from build123d import *

# Parameters (mm, degrees)
BOSS_EXTRUDE3_DEPTH = 12.7
SKETCH2_R           = 2.38125
CUT_EXTRUDE1_DEPTH  = 7.63575
SKETCH3_R           = 2.38125
CUT_EXTRUDE2_DEPTH  = 7.63575


with BuildPart() as part:
    # Sketch1 → Boss-Extrude3 (new body)
    with BuildSketch(Plane.XY):
        with BuildLine():
            Line((51.176153738, -2.63525), (68.859545977, -2.63525))
            Line((68.859545977, -2.63525), (68.859545977, -9.271))
            Line((68.859545977, -9.271), (56.159545977, -9.271))
            ThreePointArc((56.159545977, -9.271), (40.248267325, -40.248267325), (9.271, -56.159545977))
            Line((9.271, -56.159545977), (9.271, -68.956153738))
            Line((9.271, -68.956153738), (2.63525, -68.956153738))
            Line((2.63525, -68.956153738), (2.63525, -51.176153738))
            ThreePointArc((2.63525, -51.176153738), (36.234950351, -36.234950351), (51.176153738, -2.63525))
        make_face()
    extrude(amount=BOSS_EXTRUDE3_DEPTH)

    # Sketch2 → Cut-Extrude1 (cut, through all)
    with BuildSketch(Plane(origin=(9.271, 0, 0), x_dir=(0, 0, -1), z_dir=(1, 0, 0))):
        with Locations((-6.35, -62.606153738)):
            Circle(SKETCH2_R)
    extrude(amount=-CUT_EXTRUDE1_DEPTH, mode=Mode.SUBTRACT)

    # Sketch3 → Cut-Extrude2 (cut, through all)
    with BuildSketch(Plane.XZ.offset(9.271)):
        with Locations((62.509545977, 6.35)):
            Circle(SKETCH3_R)
    extrude(amount=-CUT_EXTRUDE2_DEPTH, mode=Mode.SUBTRACT)


solid = part.part
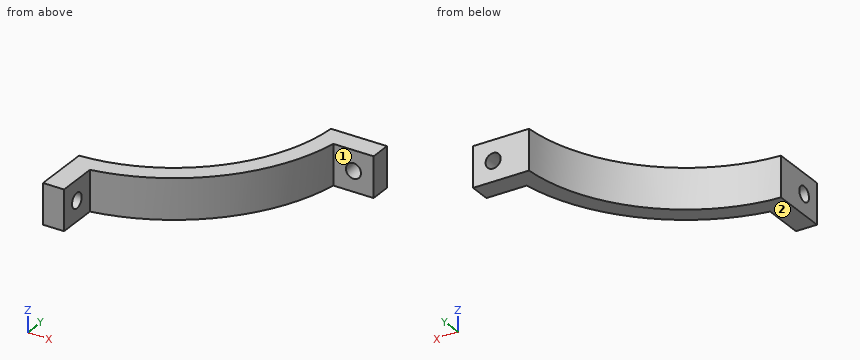
Could you check a few things on this model? Use its own coordinates, in mm. Face numbers are marked on the shaded views. A direction names the side the tool comes from. Coordinates: 2 decimals unless noted, no trailing zeros. Loops run counter-clockwise (first coordinate to the right, second up) from the corner with the lowest first, then second, coordinate; pieces in that order, holes last. Notation, with made-up numbers: (8.25, 82) -> (58.25, 82) arc R26 ccw to (58.25, 113) -> close; hole circle Ø1 at (88.25, 5). An arc over 180 degrees is marked (long way). Answer in a Markdown table with one row per item.
(1) If I drill on probe 1 along Y at (x, z) = (5.5, 6.35); probe 2 along X at (y, z) = (-56.5, 4.5); probe 3 along Y at (x, z) = (24, 11.25), over which ranges is the centre line in solid material (lowest first)?
Results found:
| item | result |
|---|---|
| probe 1 | y = -68.96 to -64.99, -60.22 to -50.95 |
| probe 2 | x = 2.64 to 9.27 |
| probe 3 | y = -51.61 to -45.28 |
(2) For the marked faces 1 and 2, which set-ups out of +Z, -Z, +X, -X, +Y, -Y let a thin tool reach every point of the face, with its end or its side?
Results found:
| item | result |
|---|---|
| face 1 | +Z, -Z, +X, -Y |
| face 2 | -Z, +X, -X, +Y, -Y |
(3) Imagine slicing it at B-B (z = 11). List the corners of the cut face in (x, y) for me.
Results found:
| item | result |
|---|---|
| outline | (2.64, -68.96) -> (9.27, -68.96) -> (9.27, -56.16) arc R56.92 ccw to (56.16, -9.27) -> (68.86, -9.27) -> (68.86, -2.64) -> (51.18, -2.64) arc R51.24 cw to (2.64, -51.18) -> close |
(4) Will these pins go through, and if not, where does the flat tip stop? pin 1 Ø3 at (x, z) = (43.5, 7.5) entering from +Y; pin 2 Ø4 at (y, z) = (-62.61, 6.35) entering from -X; pin 3 Ø1.5 at (x, z) = (41.5, 3) entering from -Y; pin 4 Ø6 at (x, z) = (11.5, 3) entering from +Y.
Results found:
| item | result |
|---|---|
| pin 1 | stops at y = -24.51 |
| pin 2 | passes through |
| pin 3 | stops at y = -39.74 |
| pin 4 | stops at y = -49.15 |
(5) Imagine slicing it at A-A (z = 6.35). List the corners of the cut face in (x, y) for me.
Results found:
| item | result |
|---|---|
| outline | (2.64, -68.96) -> (9.27, -68.96) -> (9.27, -64.99) -> (2.64, -64.99) -> close; (2.64, -60.22) -> (9.27, -60.22) -> (9.27, -56.16) arc R56.92 ccw to (56.16, -9.27) -> (60.13, -9.27) -> (60.13, -2.64) -> (51.18, -2.64) arc R51.24 cw to (2.64, -51.18) -> close; (64.89, -9.27) -> (68.86, -9.27) -> (68.86, -2.64) -> (64.89, -2.64) -> close |
(6) Imagine slicing it at D-D (y = -7). List the corners of the cut face in (x, z) for me, plus the area to 3 significant figures.
Results found:
| item | result |
|---|---|
| outline | (50.76, 0) -> (68.86, 0) -> (68.86, 12.7) -> (50.76, 12.7) -> close; hole circle Ø4.76 at (62.51, 6.35) |
| area | 212 mm^2 |
(7) Imagine slicing it at C-C (x = 8.5). List the corners of the cut face in (y, z) for me, plus the area to 3 significant figures.
Results found:
| item | result |
|---|---|
| outline | (-68.96, 0) -> (-50.53, 0) -> (-50.53, 12.7) -> (-68.96, 12.7) -> close; hole circle Ø4.76 at (-62.61, 6.35) |
| area | 216 mm^2 |
